from build123d import *

# Parameters (mm, degrees)
F1_DEPTH = 3


with BuildPart() as f1:
    # F0 (on Front) → F1 (new body)
    with BuildSketch(Plane.XZ):
        with BuildLine():
            Line((-9.1093318323, 1.994954946), (-4.331072879, 1.994954946))
            ThreePointArc((-4.331072879, 1.994954946), (-7.8363542053, 5.0190767898), (-12.3592117795, 4.0311145096))
            ThreePointArc((-12.3592117795, 4.0311145096), (-13, 0), (-12.3592117795, -4.0311145096))
            ThreePointArc((-12.3592117795, -4.0311145096), (-7.8363542053, -5.0190767898), (-4.331072879, -1.994954946))
            Line((-4.331072879, -1.994954946), (-9.1093318323, -1.994954946))
            ThreePointArc((-9.1093318323, -1.994954946), (-11.1042867783, 0), (-9.1093318323, 1.994954946))
        make_face()
        with BuildLine():
            ThreePointArc((-3.4670094842, 1.994954946), (1.032463574, 3.8644558438), (4, 0))
            ThreePointArc((4, 0), (1.032463574, -3.8644558438), (-3.4670094842, -1.994954946))
            Line((-3.4670094842, -1.994954946), (-4.331072879, -1.994954946))
            ThreePointArc((-4.331072879, -1.994954946), (-7.8363542053, -5.0190767898), (-12.3592117795, -4.0311145096))
            ThreePointArc((-12.3592117795, -4.0311145096), (2.0408634039, -12.8388035489), (13, 0))
            ThreePointArc((13, 0), (2.0408634039, 12.8388035489), (-12.3592117795, 4.0311145096))
            ThreePointArc((-12.3592117795, 4.0311145096), (-7.8363542053, 5.0190767898), (-4.331072879, 1.994954946))
            Line((-4.331072879, 1.994954946), (-3.4670094842, 1.994954946))
        make_face()
        with BuildLine():
            ThreePointArc((-12.3592117795, -4.0311145096), (-13, 0), (-12.3592117795, 4.0311145096))
            ThreePointArc((-12.3592117795, 4.0311145096), (-14.2873240939, 0), (-12.3592117795, -4.0311145096))
        make_face()
    extrude(amount=F1_DEPTH)


solid = f1.part
The listing builds one solid part. Answer for the finished solid, in the listing's coordinates (mm). A direction names the side the tool comes from. Coordinates: 2 decimals unless noted, no trailing zeros. Write each loop counter-clockwise with the first axis right and the second up, starting at its lowest first coordinate (ties: lowest second). Pieces come first, ordered by that corner, then holes. Notation, with made-up numbers: M -33,53 L 14,53 A19 ccw 14,86 Z; hole C -36,-32 d11. An arc over 180 degrees is marked long. Put each result on its own line as item: value. Start each with the question number.
1. Flat-ended cylindrical pins translate along their axes: P1, Ø1.5, axis at x = -6, y = -2, coming from the +Z side; P2, Ø1.5, axis at y = -2, z = -8.5, coming from the -X side. Find the tip coordinate at first contact, or state that the pin passes through.
2. For a pull along X with two mould halves and no side action, classify faces 3 (the flat face through (5, -3, 0)), 4 (the flat face through (-6, -1, -1.995)), 5 (the cylindrical face through (-14.287, -1.479, 0.065)) as pulls with the +X half, pulls with the -X half, needs draft (parallel to the pull), parting line crosses it, or undercut.
3. A cutting plane is placed at D-D on x = 5. Write down the section's boundary in (y, z), then the cut area to 3 significant figures.
4. Consider line 1 (Z direction, x = -4.75, y = -0.7); line 2 (X direction, y = -0.5, z = -0.75); line 3 (X direction, y = -1.9, z = 1.5). Determine where each line is inside the solid, lowest interval first. Write a range as from..to.
5. A cutting plane is placed at B-B on y = -0.65. Write down the section's boundary in (x, z).
6. Which of the six approach directions +Z, -Z, +X, -X, +Y, -Y give full straight-line access (tool end or side, diameter ignored) to faces 1 (the cylindrical face through (-11.104, -1.479, -0.044)), 2 (the flat face through (5, 0, 0))?
7. A cutting plane is placed at C-C on z = 3.25. Write down the section's boundary in (x, y).
8. A cutting plane is placed at A-A on x = -5. Write down the section's boundary in (y, z).
Resolved:
1. P1: stops at z = 11.89
1. P2: stops at x = -10.44
2. face 3: needs draft
2. face 4: undercut
2. face 5: pulls with the -X half
3. outline: M -3,-12 L 0,-12 L 0,12 L -3,12 Z
3. area: 72.0 mm2
4. line 1: z = -12.1..-1.99, 1.99..12.1
4. line 2: x = -14.23..-10.96, 3.93..12.98
4. line 3: x = -14.07..-10.42, 3.71..12.91
5. outline: M -12.36,-4.03 A13 ccw long -12.36,4.03 A5.18 ccw Z; hole M -9.11,-1.99 L -3.47,-1.99 A4 ccw long -3.47,1.99 L -9.11,1.99 A1.99 ccw Z
6. face 1: +Y, -Y
6. face 2: +Z, -Z, +X, -X, +Y
7. outline: M -13.14,-3 L -2.33,-3 L -2.33,0 L -13.14,0 Z; M 2.33,-3 L 12.59,-3 L 12.59,0 L 2.33,0 Z
8. outline: M -3,-12 L 0,-12 L 0,-1.99 L -3,-1.99 Z; M -3,1.99 L 0,1.99 L 0,12 L -3,12 Z
